Source: CAD feature listing. Evaluate the final solid. Frame: model axes, mm. A direction names the side the tool comes from. Give positions to 0.01 mm unless a question says otherwise; leave off trailing zeros. Write each loop counter-clockwise with the first axis right and the second up, starting at its lowest first coordinate (ties: lowest second). Pieces come first, ordered by that corner, then holes. Notation, with made-up numbers: M 81,-2 L 136,-2 A15 cw 136,23 Z; hole C 35.25,9.5 d4. An arc over 180 degrees is marked long. Return JSON: item names as keys, results as strings.
```python
from build123d import *

# Parameters (mm, degrees)
F0_W     = 114.3
F0_H     = 63.5
F1_DEPTH = 36.5125
F2_W     = 57.15
F2_H     = 9.525
F3_DEPTH = 63.501
F4_W     = 98.425
F4_H     = 63.5
F5_DEPTH = 19.05
F6_W     = 15.875
F6_H     = 15.875
F7_DEPTH = 19.05
F8_R     = 9.525
F9_DEPTH = 17.4635


with BuildPart() as f1:
    # F0 (on Top) → F1 (new body)
    with BuildSketch(Plane.XY):
        with Locations((-2.143128, -16.985219)):
            Rectangle(F0_W, F0_H)
    extrude(amount=F1_DEPTH)

    # F2 (on face) → F3 (cut, through all)
    with BuildSketch(Plane.XZ.offset(48.735219)):
        with Locations((26.431872, 4.7625)):
            Rectangle(F2_W, F2_H)
    extrude(amount=-F3_DEPTH, mode=Mode.SUBTRACT)

    # F4 (on face) → F5 (cut)
    with BuildSketch(Plane.XY.offset(36.5125)):
        with Locations((5.794372, -16.985219)):
            Rectangle(F4_W, F4_H)
    extrude(amount=-F5_DEPTH, mode=Mode.SUBTRACT)

    # F6 (on face) → F7 (join)
    with BuildSketch(Plane.XY.offset(17.4625)):
        with Locations((47.069372, 6.827281)):
            Rectangle(F6_W, F6_H)
        with Locations((47.069372, -40.797719)):
            Rectangle(F6_W, F6_H)
    extrude(amount=F7_DEPTH)

    # F8 (on face) → F9 (cut, through all)
    with BuildSketch(Plane.XY.offset(17.4625)):
        with Locations((-22.780628, -16.985219)):
            Circle(F8_R)
        with Locations((18.494372, -16.985219)):
            Circle(F8_R)
    extrude(amount=-F9_DEPTH, mode=Mode.SUBTRACT)


solid = f1.part
```
1) Set-up query: faces 5 (the face through (47, -32.86, 27)), 6 (the face through (39.132, -41, 27)), 7 (the face through (32, -17, 9.525)). Return all of +Z, -Z, +X, -X, +Y, -Y with unobstructed straight access to the full face (end or side cutting, diameter ignored); none if empty.
Numbers:
{"face 5": "+Z, +X", "face 6": "+Z, +Y, -Y", "face 7": "-Z, +X, +Y, -Y"}
2) Cut plane D-D, the plane y = -11. Return the cut outline in (x, z) (1 decimal).
Numbers:
{"outline": "M -59.3,0 L -30.2,0 L -30.2,17.5 L -43.4,17.5 L -43.4,36.5 L -59.3,36.5 Z; M -15.4,0 L -2.1,0 L -2.1,9.5 L 11.1,9.5 L 11.1,17.5 L -15.4,17.5 Z; M 25.9,9.5 L 55,9.5 L 55,17.5 L 25.9,17.5 Z"}
3) Draft query along X for faces 1 (the face through (47, 7, 36.512)), 2 (the face through (-43.418, -17, 27)), 3 (the face through (5, -17, 17.463)), 4 (the face through (-59.293, -17, 18)). Return one class per face: released by +X, released by -X, zero draft, split by the parting line, or undercut.
Numbers:
{"face 1": "zero draft", "face 2": "undercut", "face 3": "undercut", "face 4": "released by -X"}
4) Contact query for flat-ended pins moving along their axis: pin 1 Ø5 at (x, y) = (6, -5.5) entering from +Z; pin 2 Ø3 at (y, z) = (-25.5, 4.5) entering from +X. Output: stop coordinate, or through.
Numbers:
{"pin 1": "stops at z = 17.46", "pin 2": "stops at x = -2.14"}
5) Cut plane A-A, the plane x = -22.5. Return the cut outline in (y, z).
Numbers:
{"outline": "M -48.74,0 L -26.51,0 L -26.51,17.46 L -48.74,17.46 Z; M -7.46,0 L 14.76,0 L 14.76,17.46 L -7.46,17.46 Z"}
6) Line query: line 1 (X direction, y = 3, z = 30.5); line 2 (X direction, y = -21.5, z = 12); line 3 (X direction, y = -4, z = 2.5). Output: solid intervals per line, ascending. Write a range as [from, to].
Numbers:
{"line 1": "x = [-59.29, -43.42], [39.13, 55.01]", "line 2": "x = [-59.29, -31.17], [-14.39, 10.11], [26.88, 55.01]", "line 3": "x = [-59.29, -2.14]"}
7) Cut plane C-C, the plane y = -3. Return the cut outline in (x, z) (1 decimal), then the cut area to 3 significant figures.
Numbers:
{"outline": "M -59.3,0 L -2.1,0 L -2.1,9.5 L 55,9.5 L 55,17.5 L -43.4,17.5 L -43.4,36.5 L -59.3,36.5 Z", "area": "1,750 mm²"}
8) Cut plane B-B, the plane z = 25.5. Return the cut outline in (x, y), then the cut area to 3 significant figures.
Numbers:
{"outline": "M -59.29,-48.74 L -43.42,-48.74 L -43.42,14.76 L -59.29,14.76 Z; M 39.13,-48.74 L 55.01,-48.74 L 55.01,-32.86 L 39.13,-32.86 Z; M 39.13,-1.11 L 55.01,-1.11 L 55.01,14.76 L 39.13,14.76 Z", "area": "1,510 mm²"}
